Check sheet for the modelled part. Datum: model origin and axes. Units: mm. A direction names the side the tool comes from. Round coordinates to 2 decimals unless told otherwise and drop trailing zeros. Write each loop counter-clockwise with the first axis right and the second up, starting at its lowest first coordinate (ties: lowest second). Pieces come first, ordered by that corner, then holes.
Item 1: Tool access check on faces 1 (the flat face through (-22.268, 15, 6)), 2 (the flat face through (-31, 8, 0)). Record the directions out of +Z, -Z, +X, -X, +Y, -Y that give a thin tool (end or side, any length) a straight path to the whole face; none if there is none.
Item 2: Material ranges on line 1 (X direction, y = 11, z = 4.75); line 2 (Y direction, x = -15, z = 2.25); line 3 (Z direction, x = -38.5, y = 13), recorded low to high.
Item 3: Release check for a two-part mould opening along X. For faces 3 (the flat face through (16.8, 17.3, 8)), 4 (the flat face through (-29, 23.073, 6)) record: +X half, -X half, draft (parallel to the pull), parting line (faces both ways), or undercut.
Item 4: Cross-section at A-A on x = -46.5. Enter the section's corners in (y, z).
Item 5: Cross-section at D-D on z = 5. Enter the section's corners in (x, y).
Item 6: Cross-section at B-B on y = 21. Enter the section's corners in (x, z).
Item 7: Go/stop test with flat-tipped pins: pin 1 Ø16.5 at (x, y) = (-42, 13.5) entering from -Z; pin 2 Ø2 at (x, z) = (16.5, 6.5) entering from +Y. Record where each tip stops, or that it passes through.
Item 8: Cross-section at C-C on z = 10. Enter the section's corners in (x, y), plus the area to 3 significant figures.
from build123d import *

# Parameters (mm, degrees)
F0_R     = 3.5
F1_DEPTH = 4
F3_DEPTH = 4
F4_W     = 15
F4_H     = 15.06
F4_R     = 3.5
F5_DEPTH = 4


# Not quite as in the source:
# - a feature names something its author has since deleted; it is built from what else it names


with BuildPart() as f1:
    # F0 (on Top) → F1 (new body)
    with BuildSketch(Plane.XY):
        with BuildLine():
            Line((-74.7510943777, 23.0731565692), (-87.7510943777, 23.0731565692))
            Line((-87.7510943777, 23.0731565692), (-87.7510943777, 19.0731565692))
            Line((-87.7510943777, 19.0731565692), (-87.7510943777, 17.0731565692))
            Line((-87.7510943777, 17.0731565692), (-87.7510943777, -6.9268434308))
            Line((-87.7510943777, -6.9268434308), (-74.7510943777, -6.9268434308))
            Line((-74.7510943777, -6.9268434308), (-74.7510943777, 10.0396581329))
            ThreePointArc((-74.7510943777, 10.0396581329), (-78.2510943777, 13.5396581329), (-74.7510943777, 17.0396581329))
            Line((-74.7510943777, 17.0396581329), (-74.7510943777, 23.0731565692))
        make_face()
        Polygon((-87.7510943777, 19.0731565692), (-87.7510943777, 23.0731565692), (-89.7579597334, 23.0731565692), (-89.7579597334, -6.9268434308), (-87.7510943777, -6.9268434308), (-87.7510943777, 17.0731565692), align=None)
        with BuildLine():
            Line((30.2420402666, 23.0731565692), (-74.7510943777, 23.0731565692))
            Line((-74.7510943777, 23.0731565692), (-74.7510943777, 17.0396581329))
            ThreePointArc((-74.7510943777, 17.0396581329), (-72.2762206436, 16.0145318671), (-71.2510943777, 13.5396581329))
            ThreePointArc((-71.2510943777, 13.5396581329), (-72.2762206436, 11.0647843988), (-74.7510943777, 10.0396581329))
            Line((-74.7510943777, 10.0396581329), (-74.7510943777, -6.9268434308))
            Line((-74.7510943777, -6.9268434308), (30.2420402666, -6.9268434308))
            Line((30.2420402666, -6.9268434308), (30.2420402666, 23.0731565692))
        make_face()
        with Locations((-44.7579597334, 13.8557466809)):
            Circle(F0_R, mode=Mode.SUBTRACT)
        with Locations((-14.7579597334, 13.9075608123)):
            Circle(F0_R, mode=Mode.SUBTRACT)
        with Locations((15.2420402666, 13.9186258558)):
            Circle(F0_R, mode=Mode.SUBTRACT)
    extrude(amount=F1_DEPTH)

    # F2 (on face) → F3 (join)
    with BuildSketch(Plane.XY.offset(4)):
        Polygon((30.2420402666, 23.0731565692), (30.2320402666, 23.0731565692), (30.2420402666, -6.9268434308), align=None)
        Polygon((30.2420402666, -6.9268434308), (30.2320402666, 23.0731565692), (22.7320402666, 23.0731565692), (22.7320402666, 8.0131565692), (7.7320402666, 8.0131565692), (7.7320402666, 23.0731565692), (-7.2679597334, 23.0731565692), (-7.2679597334, 8.0131565692), (-22.2679597334, 8.0131565692), (-22.2679597334, 23.0731565692), (-37.2679597334, 23.0731565692), (-37.2679597334, 8.0131565692), (-52.2679597334, 8.0131565692), (-52.2679597334, 23.0731565692), (-67.2679597334, 23.0731565692), (-67.2679597334, 8.0131565692), (-82.2679597334, 8.0131565692), (-82.2679597334, 23.0731565692), (-89.7579597334, 23.0731565692), (-89.7579597334, -6.9268434308), align=None)
    extrude(amount=F3_DEPTH)

    # F4 (on face) → F5 (join)
    with BuildSketch(Plane.XY.offset(8)):
        Polygon((-82.2679597334, 23.0731565692), (-89.7579597334, 23.0731565692), (-89.7579597334, -6.9268434308), (30.2420402666, -6.9268434308), (30.2420402666, 23.0731565692), (22.7320402666, 23.0731565692), (22.7320402666, 8.0131565692), (7.7320402666, 8.0131565692), (7.7320402666, 23.0731565692), (-7.2679597334, 23.0731565692), (-7.2679597334, 8.0131565692), (-22.2679597334, 8.0131565692), (-22.2679597334, 23.0731565692), (-37.2679597334, 23.0731565692), (-37.2679597334, 8.0131565692), (-52.2679597334, 8.0131565692), (-52.2679597334, 23.0731565692), (-67.2679597334, 23.0731565692), (-67.2679597334, 8.0131565692), (-82.2679597334, 8.0131565692), align=None)
        with Locations((-44.7679597334, 15.5431565692)):
            Rectangle(F4_W, F4_H)
        with Locations((-44.7580007362, 13.8554783896)):
            Circle(F4_R, mode=Mode.SUBTRACT)
        with Locations((-14.7679597334, 15.5431565692)):
            Rectangle(F4_W, F4_H)
        with Locations((-14.7580007362, 13.907292521)):
            Circle(F4_R, mode=Mode.SUBTRACT)
        with Locations((15.2320402666, 15.5431565692)):
            Rectangle(F4_W, F4_H)
        with Locations((15.2419992638, 13.9183575645)):
            Circle(F4_R, mode=Mode.SUBTRACT)
        with Locations((-74.7679597334, 15.5431565692)):
            Rectangle(F4_W, F4_H)
        with Locations((-74.7511353805, 13.5393898416)):
            Circle(F4_R, mode=Mode.SUBTRACT)
    extrude(amount=F5_DEPTH)


solid = f1.part
Response values:
1. face 1: +Y
1. face 2: -Z, +X, -X, +Y, -Y
2. line 1: x = -89.76 to -82.27, -67.27 to -52.27, -37.27 to -22.27, -7.27 to 7.73, 22.73 to 30.24
2. line 2: y = -6.93 to 10.42, 17.4 to 23.07
2. line 3: z = 0 to 4, 8 to 12
3. face 3: undercut
3. face 4: draft
4. outline: (-6.93, 0) - (10.82, 0) - (10.82, 4) - (8.01, 4) - (8.01, 8) - (10.82, 8) - (10.82, 12) - (-6.93, 12) - close; (16.89, 0) - (23.07, 0) - (23.07, 4) - (16.89, 4) - close; (16.89, 8) - (23.07, 8) - (23.07, 12) - (16.89, 12) - close
5. outline: (-89.76, -6.93) - (30.24, -6.93) - (30.24, 23.07) - (22.73, 23.07) - (22.73, 8.01) - (7.73, 8.01) - (7.73, 23.07) - (-7.27, 23.07) - (-7.27, 8.01) - (-22.27, 8.01) - (-22.27, 23.07) - (-37.27, 23.07) - (-37.27, 8.01) - (-52.27, 8.01) - (-52.27, 23.07) - (-67.27, 23.07) - (-67.27, 8.01) - (-82.27, 8.01) - (-82.27, 23.07) - (-89.76, 23.07) - close
6. outline: (-89.76, 0) - (30.24, 0) - (30.24, 12) - (-89.76, 12) - close; hole (-82.27, 4) - (-67.27, 4) - (-67.27, 8) - (-82.27, 8) - close; hole (-52.27, 4) - (-37.27, 4) - (-37.27, 8) - (-52.27, 8) - close; hole (-22.27, 4) - (-7.27, 4) - (-7.27, 8) - (-22.27, 8) - close; hole (7.73, 4) - (22.73, 4) - (22.73, 8) - (7.73, 8) - close
7. pin 1: stops at z = 0
7. pin 2: stops at y = 8.01
8. outline: (-89.76, -6.93) - (30.24, -6.93) - (30.24, 23.07) - (-89.76, 23.07) - close; hole circle Ø7 at (-74.75, 13.54); hole circle Ø7 at (-44.76, 13.86); hole circle Ø7 at (-14.76, 13.91); hole circle Ø7 at (15.24, 13.92)
8. area: 3,450 mm2
